Build history of the part. All positions in model axes, mm. A direction names the side the tool comes from. Give positions to 0.01 mm unless a question says otherwise; leave off trailing zeros. Loops run counter-clockwise (first coordinate to the right, second up) from the corner with the lowest first, then second, coordinate; pieces in that order, holes last. Notation, with made-up numbers: (-9, -18) - (11, -18) arc R19 ccw to (11, -1) - close; hole circle Ø10 at (71.25, 28). An arc over 180 degrees is marked (long way). Return JSON: item names as keys, results as strings. Group by question number.
1) Drill centre lines: probe 1 along Y at (x, z) = (-55, -19); probe 2 along X at (y, z) = (-12.75, -18); probe 3 along Z at (x, y) = (-50.5, -13.75). Where is each one in solid material? Low to high. Write a range as from..to.
2) 3-axis set-ups, long thin cutter, end or side, ignore diameter. For faces 4 (the face through (-49, -10, -17)), 5 (the face through (52, -10, -17)), 6 (the face through (-58.247, -9.857, -26.93)), 7 (the face through (49, -10, -22)), 8 (the face through (24.86, -9.86, -11.18)): which of +Z, -Z, +X, -X, +Y, -Y reach the whole face in a straight line?
3) Slice it at B-B (x = 0). List the corners of the cut face in (y, z), and give its area (3 significant figures).
4) Drop flat-ended pins along their axis: pin 1 (10 mm diameter, centred on x = -33, y = -11.5, fed in from +Z); pin 2 (3.5 mm diameter, centred on y = -7, z = -2.5, fed in from -X); pin 3 (10.5 mm diameter, centred on x = 45, y = -10, fed in from +Z). Give the stop position or say it passes through.
5) Slice it at A-A (y = -10). Count the separate pieces of the cut face and the enclosed holes in it, and give its area (3 significant figures).
6) Slice it at D-D (x = 45). List the corners of the cut face in (y, z), and give its area (3 significant figures).
7) Mould opens along Z. For faces 1 (the face through (-0.358, -9.86, 29.727)), 2 (the face through (-6, -20, -21)), 3 (the face through (35.51, -9.86, -14.15)) say: released by +Z, released by -Z, zero draft, split by the parting line, or undercut.
8) Slice it at C-C (z = -19). List the corners of the cut face in (x, y), and give its area (3 significant figures).
```python
from build123d import *

# Parameters (mm, degrees)
F0_R     = 2.75
F0_R_2   = 21.25
F1_DEPTH = 20
F2_R     = 3.25
F3_DEPTH = 25
F4_R     = 5.5
F5_DEPTH = 22


with BuildPart() as f1:
    # F0 (on Front) → F1 (new body)
    with BuildSketch(Plane.XZ):
        with BuildLine():
            Line((32.5, -7), (32.5, 0))
            ThreePointArc((32.5, 0), (0, 32.5), (-32.5, 0))
            Line((-32.5, 0), (-32.5, -7))
            ThreePointArc((-32.5, -7), (-35.428932, -14.071068), (-42.5, -17))
            Line((-42.5, -17), (-65, -17))
            Line((-65, -17), (-65, -32))
            Line((-65, -32), (-32.5, -32))
            Line((-32.5, -32), (32.5, -32))
            Line((32.5, -32), (55, -32))
            Line((55, -32), (55, -17))
            Line((55, -17), (42.5, -17))
            ThreePointArc((42.5, -17), (35.428932, -14.071068), (32.5, -7))
        make_face()
        with Locations((-23.382686, -13.5)):
            Circle(F0_R, mode=Mode.SUBTRACT)
        with Locations((23.382686, -13.5)):
            Circle(F0_R, mode=Mode.SUBTRACT)
        Circle(F0_R_2, mode=Mode.SUBTRACT)
        with Locations((0, 27)):
            Circle(F0_R, mode=Mode.SUBTRACT)
    extrude(amount=F1_DEPTH)

    # F2 (on face) → F3 (cut)
    with BuildSketch(Plane.XY.offset(-17)):
        with Locations((-55, -10)):
            Circle(F2_R)
        with Locations((45, -10)):
            Circle(F2_R)
    extrude(amount=-F3_DEPTH, mode=Mode.SUBTRACT)

    # F4 (on Top) → F5 (cut)
    with BuildSketch(Plane.XY):
        with Locations((-55, -10)):
            Circle(F4_R)
        with Locations((45, -10)):
            Circle(F4_R)
    extrude(amount=-F5_DEPTH, mode=Mode.SUBTRACT)


solid = f1.part
```
Results:
{
 "1": {"probe 1": "-20..-15.5, -4.5..0", "probe 2": "-65..-59.76, -50.24..-11.29, 11.29..40.24, 49.76..55", "probe 3": "-32..-17"},
 "2": {"face 4": "+Z, -X, +Y, -Y", "face 5": "+Z, +X, +Y, -Y", "face 6": "+Z, -Z", "face 7": "+Z", "face 8": "+Y, -Y"},
 "3": {"outline": "(-20, -32) - (0, -32) - (0, -21.25) - (-20, -21.25) - close; (-20, 21.25) - (0, 21.25) - (0, 24.25) - (-20, 24.25) - close; (-20, 29.75) - (0, 29.75) - (0, 32.5) - (-20, 32.5) - close", "area": "330 mm2"},
 "4": {"pin 1": "z = 16.5", "pin 2": "x = -32.5", "pin 3": "z = -22"},
 "5": {"separate pieces": "3", "enclosed holes": "4", "area": "2,880 mm2"},
 "6": {"outline": "(-20, -32) - (-13.25, -32) - (-13.25, -22) - (-15.5, -22) - (-15.5, -17) - (-20, -17) - close; (-6.75, -32) - (0, -32) - (0, -17) - (-4.5, -17) - (-4.5, -22) - (-6.75, -22) - close", "area": "180 mm2"},
 "7": {"face 1": "undercut", "face 2": "zero draft", "face 3": "released by +Z"},
 "8": {"outline": "(-65, -20) - (-9.52, -20) - (-9.52, 0) - (-65, 0) - close; (9.52, -20) - (55, -20) - (55, 0) - (9.52, 0) - close; hole circle Ø11 at (-55, -10); hole circle Ø11 at (45, -10)", "area": "1,830 mm2"}
}
